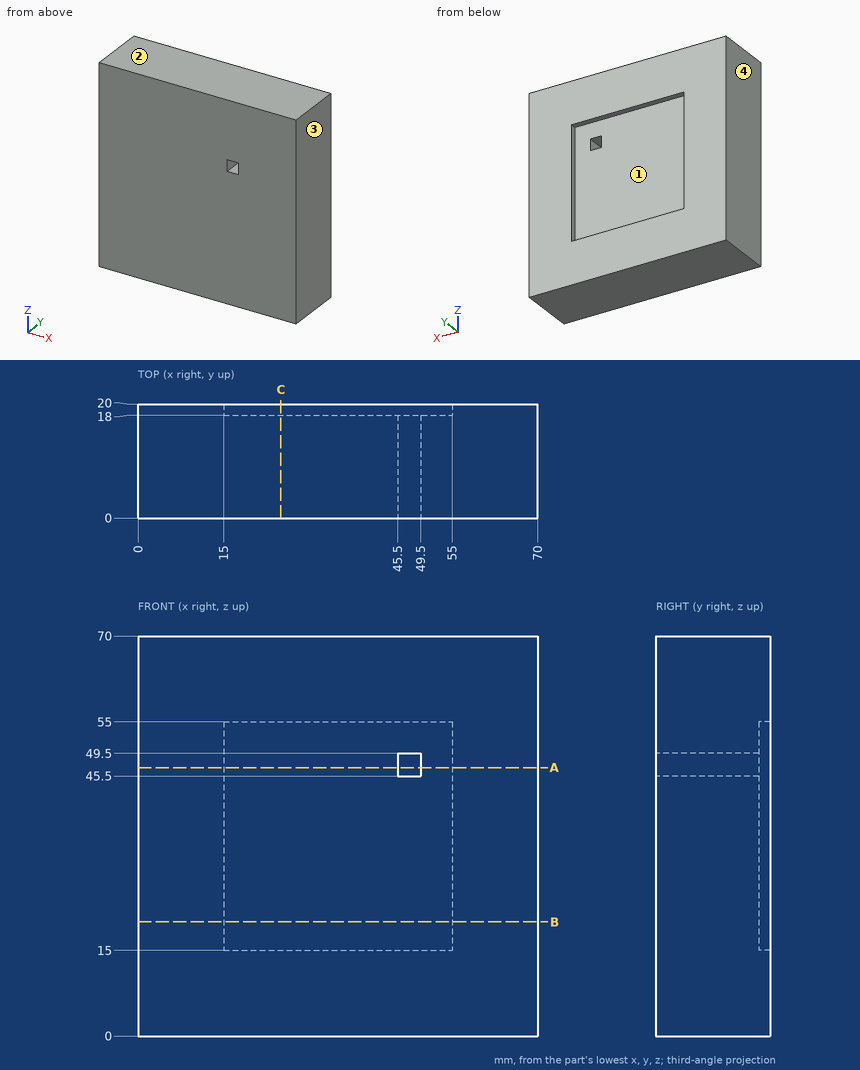
Answer from the drawing. Dimensions are ordinates in mm from the lowest x, y and z of the part. Coordinates: 2 decimals unless noted, no trailing zeros. Write each loop counter-clockwise with the first axis right and the second up, starting at its lowest first coordinate (ties: lowest second). Pieces come first, ordered by that corner, then holes. Notation, with made-up numbers: (33, 64.5) - (74, 64.5) arc R9 ccw to (74, 76.5) - close; hole circle Ø1 at (-38, 88). An arc over 180 degrees is marked (long way). Return JSON: item names as keys, results as strings. Group by question number.
Q1. A flat-ended cylindrical pin translates along its axis: pin 1 Ø6 at (x, z) = (23.5, 47) entering from +Y. Find the tip coordinate at first contact, or state that the pin passes through.
Q2. For a pull along X with two mould halves and no side action, classify the marked faces 1, 2, 3 and 4 as +X half, -X half, draft (parallel to the pull), parting line (faces both ways), or undercut.
Q3. The part is cut by section A-A on z = 47. Write down the section's boundary in (x, y).
Q4. Find the intervals of material crossed by line 1 along Z through (x, y) = (44.5, 19); line 2 along Y through (x, z) = (23.5, 17.5); line 3 along Z through (x, y) = (49, 4.5), in increasing order. Write a range as [from, to].
Q5. The part is cut by section C-C on x = 25. Write down the section's boundary in (y, z).
Q6. The part is cut by section B-B on z = 20. Write down the section's boundary in (x, y).
Evaluation:
{
 "1": {"pin 1": "stops at y = 18"},
 "2": {"face 1": "undercut", "face 2": "draft", "face 3": "+X half", "face 4": "-X half"},
 "3": {"outline": "(0, 0) - (45.5, 0) - (45.5, 18) - (15, 18) - (15, 20) - (0, 20) - close; (49.5, 0) - (70, 0) - (70, 20) - (55, 20) - (55, 18) - (49.5, 18) - close"},
 "4": {"line 1": "z = [0, 15], [55, 70]", "line 2": "y = [0, 18]", "line 3": "z = [0, 45.5], [49.5, 70]"},
 "5": {"outline": "(0, 0) - (20, 0) - (20, 15) - (18, 15) - (18, 55) - (20, 55) - (20, 70) - (0, 70) - close"},
 "6": {"outline": "(0, 0) - (70, 0) - (70, 20) - (55, 20) - (55, 18) - (15, 18) - (15, 20) - (0, 20) - close"}
}
